Here's how the part is built. I have some questions about the finished solid (model axes, mm). Face numbers are marked on the shaded views. A direction names the side the tool comes from. Round coordinates to 2 decimals unless told otherwise and drop trailing zeros. Loops run counter-clockwise (first coordinate to the right, second up) from the corner with the lowest first, then second, coordinate; pieces in that order, holes last. Notation, with made-up numbers: (42.5, -25) -> (67.5, -25) arc R34 cw to (67.5, 11) -> close; hole circle Ø2 at (59, 58). An arc over 180 degrees is marked (long way). Use one line per item in the form item = value. Start each with the question number.
Item 1: If I drill on L1, parallel to X at y = 5, z = 18; L2, parallel to Y at x = 19, z = 0; L3, parallel to X at y = -0.5, z = 17, over which ranges is the centre line in solid material (lowest first)? Write a range as [from, to].
Item 2: If we section it at B-B (x = 25): Write out the boundary of the cut face in (y, z).
Item 3: Thinking about a two-plate mould opening in Z: for the marked faces 1, 2 and 3, which applies, released by +Z, released by -Z, zero draft, split by the parting line, or undercut?
Item 4: If we section it at A-A (z = 18): Write out the boundary of the cut face in (x, y).
Item 5: If we section it at C-C (y = 0): State how many separate pieces and enclosed holes the cut face has, then the cut area to 3 significant figures.
Item 6: For the marked faces 4, 5 and 6, which set-ups out of +Z, -Z, +X, -X, +Y, -Y let a thin tool reach every point of the face, with its end or its side?
Item 7: I'm going to push flat-ended pins straight in: pin 1 Ø5 at (y, z) = (4, 6) entering from +X; pin 2 Ø7.5 at (y, z) = (-3.5, -1.5) entering from -X; pin 3 Ø13.5 at (y, z) = (3, 4) entering from -X; pin 4 Ø2 at (x, y) = (19.5, -5.5) entering from -Z. Where does each tip first touch, or does it pass through?
```python
from build123d import *

# Parameters (mm, degrees)
SKETCH1_R           = 12.5
BOSS_EXTRUDE1_DEPTH = 44
EXTRUDE_THIN1_START = 0.5
SKETCH1_4_R         = 8.5
SKETCH1_4_R_2       = 8
EXTRUDE_THIN1_DEPTH = 37.5
BOSS_EXTRUDE2_START = 0.8
SKETCH1_5_R         = 11.5
SKETCH1_5_R_2       = 8
BOSS_EXTRUDE2_DEPTH = 37
BOSS_EXTRUDE3_START = 0.3
SKETCH1_6_R         = 12.5
SKETCH1_6_R_2       = 11.5
BOSS_EXTRUDE3_DEPTH = 39
BOSS_EXTRUDE4_START = 1
BOSS_EXTRUDE4_DEPTH = 1
FILLET1_R           = 0.5
SKETCH4_R           = 2.15
CUT_EXTRUDE3_DEPTH  = 64.647152332
CHAMFER1_SIZE       = 1


with BuildPart() as part:
    # Sketch1 → Boss-Extrude1 (new body)
    with BuildSketch(Plane(origin=(0, 0, 0), x_dir=(0, 0, -1), z_dir=(1, 0, 0))):
        Polygon((-25, -10), (-23.5, -8.5), (-23.5, 13.5), (-12.5, 13.5), (-7.5, 19.6), (7.5, 19.6), (12.5, 13.5), (23.5, 13.5), (23.5, -8.5), (25, -10), (25, -19), (10, -19), (8.5, -17.5), (-8.5, -17.5), (-10, -19), (-25, -19), align=None)
        Circle(SKETCH1_R, mode=Mode.SUBTRACT)
    extrude(amount=BOSS_EXTRUDE1_DEPTH)



with BuildPart() as body_2:
    # Sketch1_4 → Extrude-Thin1 (new body)
    with BuildSketch(Plane(origin=(0, 0, 0), x_dir=(0, 0, -1), z_dir=(1, 0, 0)).offset(EXTRUDE_THIN1_START)):
        Circle(SKETCH1_4_R)
        Circle(SKETCH1_4_R_2, mode=Mode.SUBTRACT)
    extrude(amount=EXTRUDE_THIN1_DEPTH)

    # Sketch1_5 → Boss-Extrude2 (add)
    with BuildSketch(Plane(origin=(0, 0, 0), x_dir=(0, 0, -1), z_dir=(1, 0, 0)).offset(BOSS_EXTRUDE2_START)):
        Circle(SKETCH1_5_R)
        Circle(SKETCH1_5_R_2, mode=Mode.SUBTRACT)
    extrude(amount=BOSS_EXTRUDE2_DEPTH)


with BuildPart() as part_1:
    add(part.part)

    add(body_2.part)  # Boss-Extrude3 merges body 2
    # Sketch1_6 → Boss-Extrude3 (add)
    with BuildSketch(Plane(origin=(0, 0, 0), x_dir=(0, 0, -1), z_dir=(1, 0, 0)).offset(BOSS_EXTRUDE3_START)):
        Circle(SKETCH1_6_R)
        Circle(SKETCH1_6_R_2, mode=Mode.SUBTRACT)
    extrude(amount=BOSS_EXTRUDE3_DEPTH)

    # Sketch3 → Boss-Extrude4 (add)
    with BuildSketch(Plane(origin=(39.3, 0, 0), x_dir=(0, 0, -1), z_dir=(1, 0, 0)).offset(BOSS_EXTRUDE4_START)):
        with BuildLine():
            Line((-1.008608766, -11.455684543), (-1.096313876, -12.451831025))
            ThreePointArc((-1.096313876, -12.451831025), (0, 12.5), (1.096313876, -12.451831025))
            Line((1.096313876, -12.451831025), (1.008608766, -11.455684543))
            ThreePointArc((1.008608766, -11.455684543), (1.561971623, -10.425790507), (2.714072041, -10.624679428))
            ThreePointArc((2.714072041, -10.624679428), (4.353799231, -10.302975473), (3.408913328, -8.924792132))
            ThreePointArc((3.408913328, -8.924792132), (0, 9.553669697), (-3.408913328, -8.924792132))
            ThreePointArc((-3.408913328, -8.924792132), (-4.353799231, -10.302975473), (-2.714072041, -10.624679428))
            ThreePointArc((-2.714072041, -10.624679428), (-1.561971623, -10.425790507), (-1.008608766, -11.455684543))
        make_face()
    extrude(amount=BOSS_EXTRUDE4_DEPTH)

    # Fillet1
    fillet1_edges = [part_1.edges().sort_by_distance(p)[0] for p in [
        (44, -9.25, 24.25),
        (44, -14.5, 25),
        (0, 2.5, 23.5),
        (0, 13.5, 18),
        (0, 16.55, 10),
        (0, 19.6, 0),
        (0, 16.55, -10),
        (0, 13.5, -18),
        (0, 2.5, -23.5),
        (0, -9.25, -24.25),
        (0, -14.5, -25),
        (0, -14.5, 25),
        (0, -9.25, 24.25),
        (22, -8.5, 23.5),
        (22, 13.5, 23.5),
        (22, 13.5, 12.5),
        (22, 19.6, 7.5),
        (22, 19.6, -7.5),
        (22, 13.5, -12.5),
        (22, 13.5, -23.5),
        (22, -8.5, -23.5),
        (22, -10, -25),
        (22, -10, 25),
        (44, -14.5, -25),
        (44, -9.25, -24.25),
        (44, 2.5, -23.5),
        (44, 13.5, -18),
        (44, 16.55, -10),
        (44, 19.6, 0),
        (44, 16.55, 10),
        (44, 13.5, 18),
        (44, 2.5, 23.5),
    ]]
    fillet(fillet1_edges, radius=FILLET1_R)

    # Sketch4 → Cut-Extrude3 (cut, through all)
    with BuildSketch(Plane.XZ.offset(19)):
        with Locations(Location((5, 18, 0), (0, 0, 270))):
            Circle(SKETCH4_R)
        with Locations(Location((39, 18, 0), (0, 0, 270))):
            Circle(SKETCH4_R)
        with Locations(Location((39, -18, 0), (0, 0, 270))):
            Circle(SKETCH4_R)
        with Locations(Location((5, -18, 0), (0, 0, 270))):
            Circle(SKETCH4_R)
    extrude(amount=-CUT_EXTRUDE3_DEPTH, mode=Mode.SUBTRACT)

    # Chamfer1
    chamfer1_edges = [part_1.edges().sort_by_distance(p)[0] for p in [
        (5, 13.5, -15.85),
        (39, 13.5, -15.85),
        (39, 13.5, 20.15),
        (39, -19, 20.15),
        (5, 13.5, 20.15),
        (5, -19, 20.15),
    ]]
    chamfer(chamfer1_edges, length=CHAMFER1_SIZE)


solid = part_1.part
```
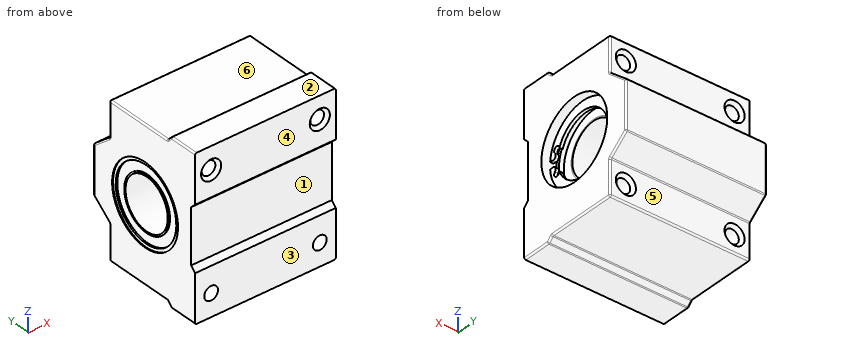
Values found:
q1.L1 = [0, 2.85], [7.15, 36.85], [41.15, 44]
q1.L2 = [-17.5, -8], [8, 19.6]
q1.L3 = [0, 3.1], [6.9, 37.1], [40.9, 44]
q2.outline = (-19, -25) -> (-10.21, -25) arc R0.5 ccw to (-9.85, -24.85) -> (-8.65, -23.65) arc R0.5 cw to (-8.29, -23.5) -> (13, -23.5) arc R0.5 ccw to (13.5, -23) -> (13.5, -12.74) arc R0.5 cw to (13.68, -12.35) -> (19.42, -7.65) arc R0.5 ccw to (19.6, -7.26) -> (19.6, 7.26) arc R0.5 ccw to (19.42, 7.65) -> (13.68, 12.35) arc R0.5 cw to (13.5, 12.74) -> (13.5, 23) arc R0.5 ccw to (13, 23.5) -> (-8.29, 23.5) arc R0.5 cw to (-8.65, 23.65) -> (-9.85, 24.85) arc R0.5 ccw to (-10.21, 25) -> (-19, 25) -> (-19, 10) -> (-17.5, 8.5) -> (-17.5, -8.5) -> (-19, -10) -> close; hole circle Ø16 at (0, 0)
q3.face_1 = undercut
q3.face_2 = released by +Z
q3.face_3 = zero draft
q4.outline = (0, -19) -> (1.85, -19) -> (2.85, -18) -> (2.85, 12.5) -> (1.85, 13.5) -> (0.5, 13.5) arc R0.5 ccw to (0, 13) -> close; (7.15, -18) -> (8.15, -19) -> (35.85, -19) -> (36.85, -18) -> (36.85, 12.5) -> (35.85, 13.5) -> (8.15, 13.5) -> (7.15, 12.5) -> close; (41.15, -18) -> (42.15, -19) -> (44, -19) -> (44, 13) arc R0.5 ccw to (43.5, 13.5) -> (42.15, 13.5) -> (41.15, 12.5) -> close
q5.separate_pieces = 2
q5.enclosed_holes = 4
q5.area = 1,250 mm2
q6.face_4 = +Z, -Z, +X, -X, -Y
q6.face_5 = -Z, +X, -X, +Y
q6.face_6 = +Z, +X, -X, +Y
q7.pin_1 = 41.3
q7.pin_2 = through
q7.pin_3 = 0.3
q7.pin_4 = -23.5
